Source: CAD feature listing. Evaluate the final solid. Frame: model axes, mm. Face numbers are marked on the shaded views. Give positions to 0.01 mm unless a question says otherwise; leave off trailing zeros. Order: outer loops, then holes, each group sorted by start corner. A loop starts at its lowest first (then second) coordinate and runs counter-clockwise, first axis right, second up. Notation, with made-up numbers: (-28, -4.5) -> (-15, -4.5) arc R26 cw to (-15, 24.5) -> close; hole circle Ø11 at (-9.5, -33.5). An arc over 180 degrees is marked (long way). Answer in a Markdown table with one row per item.
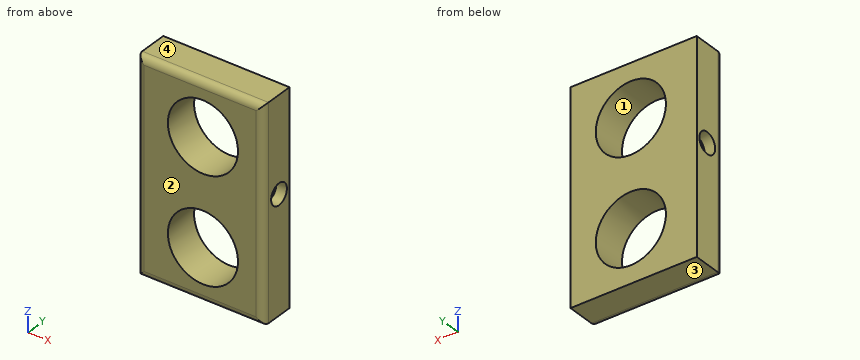
```python
from build123d import *

# Parameters (mm, degrees)
F0_W     = 36
F0_H     = 60
F1_DEPTH = 10
F2_R     = 2
F3_R     = 10
F4_DEPTH = 25
F5_R     = 3
F6_DEPTH = 3
F7_R     = 3
F8_DEPTH = 3


with BuildPart() as f1:
    # F0 (on Front) → F1 (new body)
    with BuildSketch(Plane.XZ):
        with Locations((18, 30)):
            Rectangle(F0_W, F0_H)
    extrude(amount=F1_DEPTH)

    # F2
    f2_edges = [f1.edges().sort_by_distance(p)[0] for p in [
        (0, -10, 30),
        (18, -10, 0),
        (36, -10, 30),
        (18, -10, 60),
    ]]
    fillet(f2_edges, radius=F2_R)

    # F3 (on face) → F4 (cut)
    with BuildSketch(Plane.XZ.offset(10)):
        with Locations((18.8, 15)):
            Circle(F3_R)
        with Locations((18.8, 45)):
            Circle(F3_R)
    extrude(amount=-F4_DEPTH, mode=Mode.SUBTRACT)

    # F5 (on face) → F6 (cut)
    with BuildSketch(Plane.YZ.offset(36)):
        with Locations((-4, 33)):
            Circle(F5_R)
    extrude(amount=-F6_DEPTH, mode=Mode.SUBTRACT)

    # F7 (on face) → F8 (cut)
    with BuildSketch(Plane(origin=(0, 0, 0), x_dir=(0, -1, 0), z_dir=(-1, 0, 0))):
        with Locations((4, 33)):
            Circle(F7_R)
    extrude(amount=-F8_DEPTH, mode=Mode.SUBTRACT)


solid = f1.part
```
(1) Section query C-C (y = -5.25). Return the cut outline in (x, z), plus the area to 3 significant figures.
A:
| item | result |
|---|---|
| outline | (0, 0) -> (36, 0) -> (36, 30.27) -> (33, 30.27) -> (33, 35.73) -> (36, 35.73) -> (36, 60) -> (0, 60) -> (0, 35.73) -> (3, 35.73) -> (3, 30.27) -> (0, 30.27) -> close; hole circle Ø20 at (18.8, 15); hole circle Ø20 at (18.8, 45) |
| area | 1,500 mm^2 |
(2) Pull-direction query (Z, two-part tool) for the marked faces 1, 2, 3 and 4; classes: +Z half, -Z half, draft (parallel to the pull), parting line (faces both ways), or undercut.
A:
| item | result |
|---|---|
| face 1 | undercut |
| face 2 | draft |
| face 3 | -Z half |
| face 4 | +Z half |
(3) First-contact query: pin 1 Ø3.5 at (y, z) = (-4, 33) entering from -X. Flat tip, straight axial feed; report the tip coordinate or a pass-through.
A:
| item | result |
|---|---|
| pin 1 | stops at x = 3 |
(4) Section query A-A (x = 18.8). Return the cut outline in (y, z), plus the area to 3 significant figures.
A:
| item | result |
|---|---|
| outline | (-10, 2) arc R2 ccw to (-8, 0) -> (0, 0) -> (0, 5) -> (-10, 5) -> close; (-10, 25) -> (0, 25) -> (0, 35) -> (-10, 35) -> close; (-10, 55) -> (0, 55) -> (0, 60) -> (-8, 60) arc R2 ccw to (-10, 58) -> close |
| area | 198 mm^2 |
(5) Section query D-D (z = 33). Return the cut outline in (x, y), plus the area to 3 significant figures.
A:
| item | result |
|---|---|
| outline | (0, -8) arc R2 ccw to (2, -10) -> (34, -10) arc R2 ccw to (36, -8) -> (36, -7) -> (33, -7) -> (33, -1) -> (36, -1) -> (36, 0) -> (0, 0) -> (0, -1) -> (3, -1) -> (3, -7) -> (0, -7) -> close |
| area | 322 mm^2 |
(6) Ray query, probe 1 along Z at (x, y) = (18.8, -4.5); probe 2 along Z at (x, y) = (33.8, -4); probe 3 along X at (y, z) = (-1.75, 39). Return the intervals inside material, ascending.
A:
| item | result |
|---|---|
| probe 1 | z = 0 to 5, 25 to 35, 55 to 60 |
| probe 2 | z = 0 to 30, 36 to 60 |
| probe 3 | x = 0 to 10.8, 26.8 to 36 |
(7) Section query B-B (z = 15). Return the cut outline in (x, y).
A:
| item | result |
|---|---|
| outline | (0, -8) arc R2 ccw to (2, -10) -> (8.8, -10) -> (8.8, 0) -> (0, 0) -> close; (28.8, -10) -> (34, -10) arc R2 ccw to (36, -8) -> (36, 0) -> (28.8, 0) -> close |
